```python
from build123d import *

# Parameters (mm, degrees)
EXTRUDE1_DEPTH           = 3.683
EXTRUDE1_DEPTH_BACK      = 3.683
BOSS_EXTRUDE1_DEPTH      = 7.62
BOSS_EXTRUDE1_DEPTH_BACK = 7.62
SKETCH4_R                = 1.5875


with BuildPart() as part:
    # Sketch1 → Extrude1 (new, two sides: drawn at the far end of the back side and taken through both)
    with BuildSketch(Plane.XY.offset(-EXTRUDE1_DEPTH_BACK)):
        Polygon((-12.7, 4.445), (12.7, 4.445), (15.875, 4.445), (15.875, -4.445), (12.7, -4.445), (-12.7, -4.445), align=None)
    extrude(amount=EXTRUDE1_DEPTH + EXTRUDE1_DEPTH_BACK)

    # Sketch4 → Boss-Extrude1 (add, two sides: drawn at the far end of the back side and taken through both)
    with BuildSketch(Plane.XY.offset(-BOSS_EXTRUDE1_DEPTH_BACK)):
        with Locations((12.7, 0)):
            Circle(SKETCH4_R)
    extrude(amount=BOSS_EXTRUDE1_DEPTH + BOSS_EXTRUDE1_DEPTH_BACK)


solid = part.part
```
CAD build for the part. Positions are in the model's coordinates, mm. A direction names the side the tool comes from. Coordinates: 2 decimals unless noted, no trailing zeros. Order: outer loops, then holes, each group sorted by start corner. A loop starts at its lowest first (then second) coordinate and runs counter-clockwise, first axis right, second up.
(1) Saw through at B-B, the plane x = 12.7. Write the cut outline in (y, z) (1 decimal).
Solution:
outline: (-4.4, -3.7) - (-1.6, -3.7) - (-1.6, -7.6) - (1.6, -7.6) - (1.6, -3.7) - (4.4, -3.7) - (4.4, 3.7) - (1.6, 3.7) - (1.6, 7.6) - (-1.6, 7.6) - (-1.6, 3.7) - (-4.4, 3.7) - close
(2) Drill centre lines: L1, parallel to Z at x = -3, y = 2.25; L2, parallel to X at y = -1, z = -4.5. Where is each one in solid material? Low to high.
Solution:
L1: z = -3.68 to 3.68
L2: x = 11.47 to 13.93
(3) Saw through at C-C, the plane z = -6.25. Write the cut outline in (x, y) (1 decimal), and give its area (3 significant figures).
Solution:
outline: circle Ø3.2 at (12.7, 0)
area: 7.92 mm2
(4) Saw through at D-D, the plane x = 0. Write the cut outline in (y, z) (3 decimals).
Solution:
outline: (-4.445, -3.683) - (4.445, -3.683) - (4.445, 3.683) - (-4.445, 3.683) - close
(5) Which spindle directions (+Z, -Z, +X, -X, +Y, -Y) get a long thin tool onto all of the face, cutting with end or side? Do faces 1 (the face through (13, 0, -7.62)), 2 (the face through (14.214, 0.477, 5.624)), 3 (the face through (14.214, 0.477, -5.679)). Say none if no direction does.
Solution:
face 1: -Z, +X, -X, +Y, -Y
face 2: +Z
face 3: -Z
(6) Saw through at A-A, the plane y = 0. Write the cut outline in (x, z) (1 decimal).
Solution:
outline: (-12.7, -3.7) - (11.1, -3.7) - (11.1, -7.6) - (14.3, -7.6) - (14.3, -3.7) - (15.9, -3.7) - (15.9, 3.7) - (14.3, 3.7) - (14.3, 7.6) - (11.1, 7.6) - (11.1, 3.7) - (-12.7, 3.7) - close
(7) Pin check, flat tips, straight feed: pin 1 Ø1.5 at (x, y) = (0, 3) entering from -Z; pin 2 Ø1.5 at (x, z) = (6, 5.5) entering from +Y. Stop position of each tip, or through.
Solution:
pin 1: stops at z = -3.68
pin 2: passes through
